Model file for the job. Use its own axes, mm. A direction names the side the tool comes from. Give positions to 0.01 mm unless a question says otherwise; leave off trailing zeros. Return JSON: item names as keys, results as strings. Group by question number.
1. Wall check: probe 1 along X at (y, z) = (56.25, 76); probe 2 along X at (y, z) = (45, 58.5); probe 3 along X at (y, z) = (45.25, 16). Give the ranges that are in metal, low to high. Write a range as [from, to].
2. Pin check, flat tips, straight feed: pin 1 (10.5 mm diameter, centred on x = 42.09, z = 37.95, fed in from +Y); pin 2 (1 mm diameter, centred on y = 48, z = 46, fed in from +X); pin 3 (3 mm diameter, centred on x = 40.5, z = 38, fed in from +Y). Stop position of each tip, or through.
3. 3-axis set-ups, long thin cutter, end or side, ignore diameter. For faces 1 (the face through (42.323, 52.611, 29.224)), 2 (the face through (65.05, 46.68, 56.42)), 3 (the face through (49.391, 56.843, 49.994)), 4 (the face through (13.329, 43.314, 13.832)): which of +Z, -Z, +X, -X, +Y, -Y reach the whole face in a straight line?
4. Two-plate mould, pull along Z, no slides. Class faces 5 (the face through (10.7, 43.3, 18.2)), 6 (the face through (-13.77, 47.35, 74.68)), 7 (the face through (16.587, 53, 79)), 8 (the face through (15.37, 44.3, 15.24)): released by +Z, released by -Z, zero draft, split by the parting line, or undercut.
from build123d import *

# Parameters (mm, degrees)
SKETCH1_R                      = 20
BOSS_EXTRUDE1_DEPTH            = 7.5
CHAMFER2_SIZE                  = 6
CBORE_FOR_M3_SHCS1_D           = 3.6
CBORE_FOR_M3_SHCS1_CBORE_D     = 6.5
CBORE_FOR_M3_SHCS1_CBORE_DEPTH = 3
CUT_EXTRUDE1_REACH             = 61.617
SKETCH4_R                      = 1.5
CUT_EXTRUDE2_START             = -3.5
CUT_EXTRUDE2_DEPTH             = 10
SKETCH7_R                      = 1.5
CUT_EXTRUDE3_DEPTH             = 10
CUT_EXTRUDE4_START             = -3.5
CUT_EXTRUDE4_DEPTH             = 10
SKETCH9_R                      = 1.5
CUT_EXTRUDE5_DEPTH             = 10
CUT_EXTRUDE6_START             = -3.5
CUT_EXTRUDE6_DEPTH             = 10
SKETCH11_W                     = 3
SKETCH11_H                     = 14
BOSS_EXTRUDE2_DEPTH            = 15.25
CUT_EXTRUDE7_START             = -60.310889132
SKETCH12_R                     = 2.25
CUT_EXTRUDE7_DEPTH             = 97.621778265
FILLET1_R                      = 4.25
FILLET1_OF_MIRROR4_R           = 4.25
FILLET1_OF_MIRROR5_R           = 4.25


with BuildPart() as part:
    # Sketch1 → Boss-Extrude1 (new body)
    with BuildSketch(Plane(origin=(0, 42.804564232, 0), x_dir=(1, 0, 0), z_dir=(0, 1, 0))):
        Polygon((72.89779828, -65.265836883), (37.89779828, -4.644058618), (12.276020015, -4.644058618), (-22.723979985, -65.265836883), (-9.913090852, -87.454947751), (60.086909148, -87.454947751), align=None)
        with Locations((25.086909148, -52.454947751)):
            Circle(SKETCH1_R, mode=Mode.SUBTRACT)
    extrude(amount=BOSS_EXTRUDE1_DEPTH)

    # Chamfer2
    chamfer2_edges = [part.edges().sort_by_distance(p)[0] for p in [
        (-16.318535418, 50.304564232, 76.360392317),
        (25.086909148, 50.304564232, 87.454947751),
        (66.492353714, 50.304564232, 76.360392317),
        (55.39779828, 50.304564232, 34.954947751),
        (25.086909148, 50.304564232, 4.644058618),
        (-5.223979985, 50.304564232, 34.954947751),
    ]]
    chamfer(chamfer2_edges, length=CHAMFER2_SIZE)

    # CBORE for M3 SHCS1 (through all)
    with Locations(Plane(origin=(0, 50.304564232, 0), x_dir=(1, 0, 0), z_dir=(0, 1, 0))):
        with Locations((8.086909148, -37.954947751), (42.086909148, -37.954947751), (42.086909148, -66.954947751), (8.086909148, -66.954947751)):
            CounterBoreHole(CBORE_FOR_M3_SHCS1_D / 2, CBORE_FOR_M3_SHCS1_CBORE_D / 2, CBORE_FOR_M3_SHCS1_CBORE_DEPTH)

    # Sketch4 → Cut-Extrude1 (cut, up to next)
    with BuildSketch(Plane(origin=(0, 65.879755991, 65.879755991), x_dir=(1, 0, 0), z_dir=(0, 0.707106781, 0.707106781)), mode=Mode.PRIVATE) as cut_extrude1_sk1:
        with Locations((0.086909148, -26.26928811)):
            Circle(SKETCH4_R)
    cut_extrude1_tool1 = extrude(cut_extrude1_sk1.sketch, amount=-CUT_EXTRUDE1_REACH, mode=Mode.PRIVATE) & part.part
    add(cut_extrude1_tool1.solids().sort_by_distance((0.086909, 47.304564, 84.454948))[0], mode=Mode.SUBTRACT)
    # Sketch4 → Cut-Extrude1 (cut, up to next)
    with BuildSketch(Plane(origin=(0, 65.879755991, 65.879755991), x_dir=(1, 0, 0), z_dir=(0, 0.707106781, 0.707106781)), mode=Mode.PRIVATE) as cut_extrude1_sk2:
        with Locations((50.086909148, -26.26928811)):
            Circle(SKETCH4_R)
    cut_extrude1_tool2 = extrude(cut_extrude1_sk2.sketch, amount=-CUT_EXTRUDE1_REACH, mode=Mode.PRIVATE) & part.part
    add(cut_extrude1_tool2.solids().sort_by_distance((50.086909, 47.304564, 84.454948))[0], mode=Mode.SUBTRACT)

    # Sketch5 → Cut-Extrude2 (cut)
    with BuildSketch(Plane(origin=(0, 65.879755991, 65.879755991), x_dir=(1, 0, 0), z_dir=(0, 0.707106781, 0.707106781)).offset(CUT_EXTRUDE2_START)):
        Polygon((3.262335628, -26.26928811), (1.674622388, -23.51928811), (-1.500804092, -23.51928811), (-3.088517333, -26.26928811), (-1.500804092, -29.01928811), (1.674622388, -29.01928811), align=None)
        Polygon((48.499195908, -29.01928811), (46.911482667, -26.26928811), (48.499195908, -23.51928811), (51.674622388, -23.51928811), (53.262335628, -26.26928811), (51.674622388, -29.01928811), align=None)
    extrude(amount=-CUT_EXTRUDE2_DEPTH, mode=Mode.SUBTRACT)

    # Sketch7 → Cut-Extrude3 (cut)
    with BuildSketch(Plane(origin=(-13.575463373, 15.675594866, -7.837797433), x_dir=(0.790569415, 0.547722558, -0.273861279), z_dir=(-0.612372436, 0.707106781, -0.353553391))):
        with Locations((29.661607386, -34.396624037)):
            Circle(SKETCH7_R)
        with Locations((-1.961169216, -73.126457499)):
            Circle(SKETCH7_R)
    extrude(amount=-CUT_EXTRUDE3_DEPTH, mode=Mode.SUBTRACT)

    # Sketch8 → Cut-Extrude4 (cut)
    with BuildSketch(Plane(origin=(-13.575463373, 15.675594866, -7.837797433), x_dir=(0.790569415, 0.547722558, -0.273861279), z_dir=(-0.612372436, 0.707106781, -0.353553391)).offset(CUT_EXTRUDE4_START)):
        Polygon((32.795906248, -34.906039363), (31.66992343, -31.936949262), (28.535624567, -31.427533937), (26.527308523, -33.887208712), (27.653291342, -36.856298813), (30.787590204, -37.365714138), align=None)
        Polygon((1.173129647, -73.635872825), (-0.835186398, -76.0955476), (-3.96948526, -75.586132275), (-5.095468078, -72.617042174), (-3.087152034, -70.157367399), (0.047146828, -70.666782724), align=None)
    extrude(amount=-CUT_EXTRUDE4_DEPTH, mode=Mode.SUBTRACT)

    # Sketch9 → Cut-Extrude5 (cut)
    with BuildSketch(Plane(origin=(32.390645234, 37.401495491, -18.700747745), x_dir=(0.790569415, -0.547722558, 0.273861279), z_dir=(0.612372436, 0.707106781, -0.353553391))):
        with Locations((41.627055396, -73.126457499)):
            Circle(SKETCH9_R)
        with Locations((10.004278795, -34.396624037)):
            Circle(SKETCH9_R)
    extrude(amount=-CUT_EXTRUDE5_DEPTH, mode=Mode.SUBTRACT)

    # Sketch10 → Cut-Extrude6 (cut)
    with BuildSketch(Plane(origin=(32.390645234, 37.401495491, -18.700747745), x_dir=(0.790569415, -0.547722558, 0.273861279), z_dir=(0.612372436, 0.707106781, -0.353553391)).offset(CUT_EXTRUDE6_START)):
        Polygon((39.618739352, -70.666782724), (38.492756534, -73.635872825), (40.501072578, -76.0955476), (43.63537144, -75.586132275), (44.761354259, -72.617042174), (42.753038215, -70.157367399), align=None)
        Polygon((13.138577657, -33.887208712), (12.012594839, -36.856298813), (8.878295976, -37.365714138), (6.869979932, -34.906039363), (7.99596275, -31.936949262), (11.130261613, -31.427533937), align=None)
    extrude(amount=-CUT_EXTRUDE6_DEPTH, mode=Mode.SUBTRACT)

    # Sketch11 → Boss-Extrude2 (add)
    with BuildSketch(Plane(origin=(0, 42.804564232, 0), x_dir=(1, 0, 0), z_dir=(0, 1, 0))):
        with Locations((35.086909148, -80.454947751)):
            Rectangle(SKETCH11_W, SKETCH11_H)
        with Locations((15.086909148, -80.454947751)):
            Rectangle(SKETCH11_W, SKETCH11_H)
    boss_extrude2 = extrude(amount=BOSS_EXTRUDE2_DEPTH)

    # Sketch12 → Cut-Extrude7 (cut)
    with BuildSketch(Plane(origin=(36.586909148, 0, 0), x_dir=(0, 0, -1), z_dir=(1, 0, 0)).offset(CUT_EXTRUDE7_START)):
        with Locations((-82.454947751, 53.621218058)):
            Circle(SKETCH12_R)
    cut_extrude7 = extrude(amount=CUT_EXTRUDE7_DEPTH, mode=Mode.SUBTRACT)

    # Fillet1
    fillet1_edges = [part.edges().sort_by_distance(p)[0] for p in [
        (35.086909148, 58.054564232, 87.454947751),
        (35.086909148, 58.054564232, 73.454947751),
        (15.086909148, 58.054564232, 87.454947751),
        (15.086909148, 58.054564232, 73.454947751),
    ]]
    fillet(fillet1_edges, radius=FILLET1_R)

    # Mirror4: Boss-Extrude2, Cut-Extrude7 across plane
    add(boss_extrude2.mirror(Plane(origin=(28.98538594, 0, 50.204161125), x_dir=(-0.866025404, 0, 0.5), z_dir=(0.5, 0, 0.866025404))))
    add(cut_extrude7.mirror(Plane(origin=(28.98538594, 0, 50.204161125), x_dir=(-0.866025404, 0, 0.5), z_dir=(0.5, 0, 0.866025404))), mode=Mode.SUBTRACT)

    # Fillet1 of Mirror4
    fillet1_of_mirror4_edges = [part.edges().sort_by_distance(p)[0] for p in [
        (-0.223979985, 58.054564232, 26.294693713),
        (11.900375668, 58.054564232, 33.294693713),
        (-10.223979985, 58.054564232, 43.615201789),
        (1.900375668, 58.054564232, 50.615201789),
    ]]
    fillet(fillet1_of_mirror4_edges, radius=FILLET1_OF_MIRROR4_R)

    # Mirror5: Boss-Extrude2, Cut-Extrude7 across plane
    add(boss_extrude2.mirror(Plane(origin=(-16.441931366, 0, 28.478260501), x_dir=(0.866025404, 0, 0.5), z_dir=(-0.5, 0, 0.866025404))))
    add(cut_extrude7.mirror(Plane(origin=(-16.441931366, 0, 28.478260501), x_dir=(0.866025404, 0, 0.5), z_dir=(-0.5, 0, 0.866025404))), mode=Mode.SUBTRACT)

    # Fillet1 of Mirror5
    fillet1_of_mirror5_edges = [part.edges().sort_by_distance(p)[0] for p in [
        (60.39779828, 58.054564232, 43.615201789),
        (48.273442627, 58.054564232, 50.615201789),
        (50.39779828, 58.054564232, 26.294693713),
        (38.273442627, 58.054564232, 33.294693713),
    ]]
    fillet(fillet1_of_mirror5_edges, radius=FILLET1_OF_MIRROR5_R)


solid = part.part
Result:
{
 "1": {"probe 1": "x = [13.59, 16.59], [33.59, 36.59]", "probe 2": "x = [-18.01, -15.09], [-10, 6.02], [44.15, 60.17], [65.26, 68.19]", "probe 3": "x = [6.81, 9.82], [15.5, 34.67], [40.35, 43.36]"},
 "2": {"pin 1": "stops at y = 58.03", "pin 2": "stops at x = 60.13", "pin 3": "stops at y = 47.3"},
 "3": {"face 1": "-Z, +Y", "face 2": "+X, +Y", "face 3": "+Z, +Y", "face 4": "none"},
 "4": {"face 5": "undercut", "face 6": "released by +Z", "face 7": "zero draft", "face 8": "undercut"}
}
